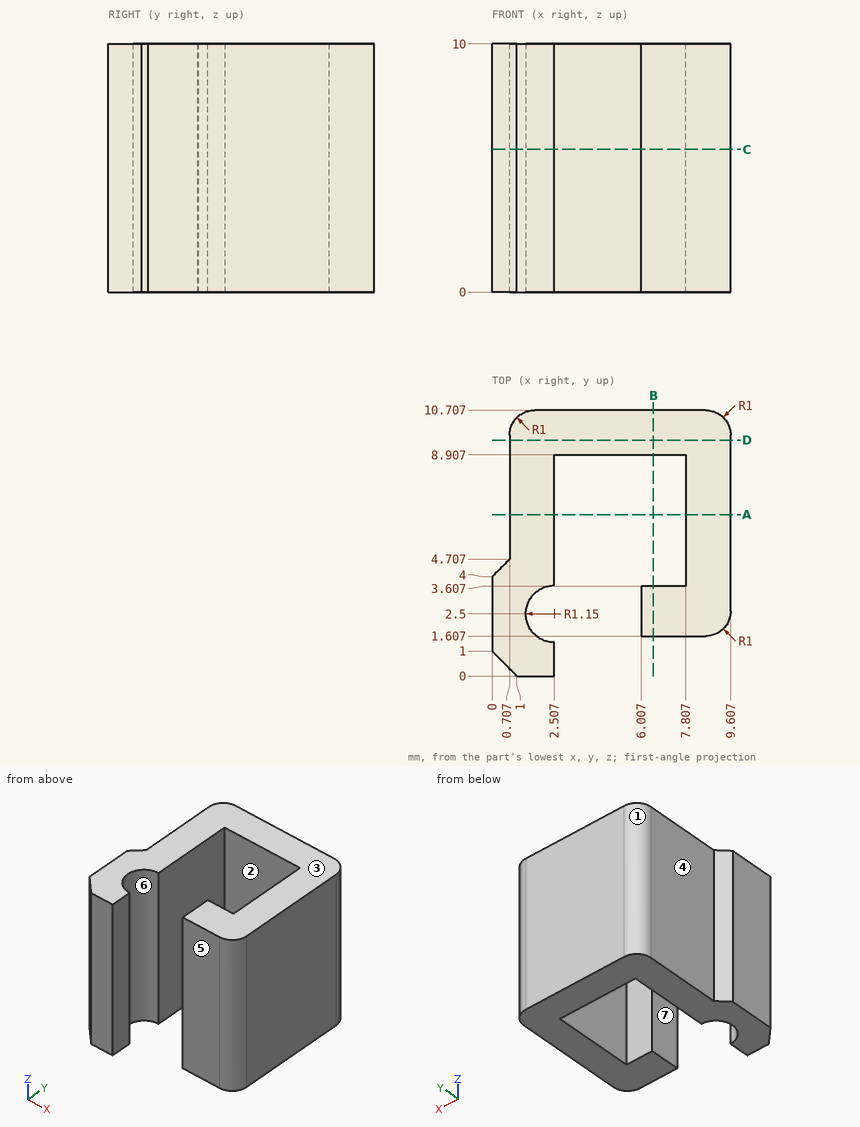
The figure shows three views and two pictorial views of one solid part (mm, origin at its lowest corner). Answer the questions. A direction names the side the tool comes from. Give positions to 0.01 mm unless a question says otherwise; leave off trailing zeros. Order: outer loops, then holes, each group sorted by start corner. A loop starts at its lowest first (then second) coordinate and runs counter-clockwise, first axis right, second up. Notation, with made-up numbers: (15, 78) -> (27, 78) arc R12 cw to (27, 98) -> close; hole circle Ø1 at (22.25, 31.25). An arc over 180 degrees is marked (long way). One line per item, written item: value.
1) Determine the mould class of the marked faces 1, 2 and 3 for opening direction Y: pulls with the +Y half, pulls with the -Y half, needs draft (parallel to the pull), parting line crosses it, or undercut.
Reported:
face 1: pulls with the +Y half
face 2: undercut
face 3: needs draft
2) Find section D-D, the plane y = 9.5. Determine the outline of the cut face in (x, z).
Reported:
outline: (0.71, 0) -> (9.61, 0) -> (9.61, 10) -> (0.71, 10) -> close
3) Flat-ended cylindrical pins translate along their axes: P1, Ø4, axis at y = 8, z = 7.5, coming from the -X side; P2, Ø0.8, axis at x = 7, z = 5.5, coming from the -Y side; P3, Ø1.1, axis at y = 1, z = 6, coming from the +X side. Find the tip coordinate at first contact, or state that the pin passes through.
Reported:
P1: stops at x = 0.71
P2: stops at y = 1.61
P3: stops at x = 2.51
4) Find the intervals of material crossed by line 1 (Y direction, x = 7.75, z = 4.5); line 2 (X direction, y = 7, z = 3); line 3 (Y direction, x = 3, z = 6), in increasing order.
Reported:
line 1: y = 1.61 to 3.61, 8.91 to 10.71
line 2: x = 0.71 to 2.51, 7.81 to 9.61
line 3: y = 8.91 to 10.71
5) Find section C-C, the plane z = 5.75. Determine the outline of the cut face in (x, y).
Reported:
outline: (0, 1) -> (1, 0) -> (2.51, 0) -> (2.51, 1.35) arc R1.15 cw to (2.51, 3.65) -> (2.51, 8.91) -> (7.81, 8.91) -> (7.81, 3.61) -> (6.01, 3.61) -> (6.01, 1.61) -> (8.61, 1.61) arc R1 ccw to (9.61, 2.61) -> (9.61, 9.71) arc R1 ccw to (8.61, 10.71) -> (1.71, 10.71) arc R1 ccw to (0.71, 9.71) -> (0.71, 4.71) -> (0, 4) -> close
6) A tool of negligible diameter and unlimited length cuts with its end or side. For the marked faces 4, 5, 6 and 7, from which of +Z, -Z, +X, -X, +Y, -Y can it reach the whole face along a straight path? Write none if from no direction.
Reported:
face 4: +Z, -Z, -X, +Y
face 5: +Z, -Z, +X, -Y
face 6: +Z, -Z
face 7: +Z, -Z, -Y
7) Find section B-B, the plane x = 6.5. Determine the outline of the cut face in (y, z), plus the area to 3 significant figures.
Reported:
outline: (1.61, 0) -> (3.61, 0) -> (3.61, 10) -> (1.61, 10) -> close; (8.91, 0) -> (10.71, 0) -> (10.71, 10) -> (8.91, 10) -> close
area: 38.0 mm^2
8) Find section A-A, the plane y = 6.5. Determine the outline of the cut face in (x, z).
Reported:
outline: (0.71, 0) -> (2.51, 0) -> (2.51, 10) -> (0.71, 10) -> close; (7.81, 0) -> (9.61, 0) -> (9.61, 10) -> (7.81, 10) -> close
